```python
from build123d import *

# Parameters (mm, degrees)
F0_W     = 117.30712
F0_H     = 72.89958
F1_DEPTH = 25.4
F2_R     = 5.08
F3_R     = 5.08
F4_W     = 25.4
F4_H     = 72.89958
F5_DEPTH = 101.6


with BuildPart() as f1:
    # F0 (on Top) → F1 (new body)
    with BuildSketch(Plane.XY):
        Rectangle(F0_W, F0_H)
    extrude(amount=F1_DEPTH)

    # F2
    f2_edges = [f1.edges().sort_by_distance(p)[0] for p in [
        (58.65356, 36.44979, 12.7),
    ]]
    fillet(f2_edges, radius=F2_R)

    # F3
    f3_edges = [f1.edges().sort_by_distance(p)[0] for p in [
        (-58.65356, 36.44979, 12.7),
    ]]
    fillet(f3_edges, radius=F3_R)

    # F4 (on face) → F5 (join)
    with BuildSketch(Plane.XY.offset(25.4)):
        with Locations((-45.95356, 0)):
            Rectangle(F4_W, F4_H)
        with Locations((45.95356, 0)):
            Rectangle(F4_W, F4_H)
    extrude(amount=F5_DEPTH)


solid = f1.part
```
CAD build for the part. Positions are in the model's coordinates, mm. A direction names the side the tool comes from. Round coordinates to 2 decimals unless told otherwise and drop trailing zeros. Order: outer loops, then holes, each group sorted by start corner. A loop starts at its lowest first (then second) coordinate and runs counter-clockwise, first axis right, second up. Notation, with made-up numbers: (-30.5, -4.5) - (-6.5, -4.5) arc R30 cw to (-6.5, 34.5) - close; hole circle Ø3 at (42.25, -29). An arc over 180 degrees is marked (long way). Use CSV: the item, a comma, the result in double quotes. Start each with the question number.
1) Pin check, flat tips, straight feed: pin 1 Ø1.5 at (x, y) = (-22, 4) entering from -Z; pin 2 Ø20 at (x, y) = (-7.5, -6) entering from +Z. Stop position of each tip, or through.
2) Wall check: L1, parallel to X at y = -4, z = 74.5; L2, parallel to Z at x = 15.5, y = 10.5. Give the ranges that are in metal, low to high. Write a range as [from, to].
3) Saw through at C-C (x = 30.5). List the corners of the cut face in (y, z), and give its area (3 significant figures).
4) Saw through at A-A (z = 89). List the corners of the cut face in (x, y), and give its area (3 significant figures).
5) Two-plate mould, pull along X, no slides. Class faces 4 (the cylindrical face through (57.205, 34.922, 12.878)), 5 (the flat face through (0, 1, 25.4)), 6 (the flat face through (-33.254, -1, 75)), 7 (the flat face through (-1, 36.45, 20)): pulls with the +X half, pulls with the -X half, needs draft (parallel to the pull), parting line crosses it, or undercut.
6) Saw through at B-B (y = 10). List the corners of the cut face in (x, z).
7) Tool access for faces 1 (the flat face through (33.254, -1, 75)), 2 (the flat face through (57.4, 35.4, 25.4)), 3 (the cylindrical face through (-57.13, 35, 12.88)): list every direction of +Z, -Z, +X, -X, +Y, -Y with a clear straight run to the whole face (end or side of a thin tool).
Values follow:
1,pin 1,"stops at z = 0"
1,pin 2,"stops at z = 25.4"
2,L1,"x = [-58.65, -33.25], [33.25, 58.65]"
2,L2,"z = [0, 25.4]"
3,outline,"(-36.45, 0) - (36.45, 0) - (36.45, 25.4) - (-36.45, 25.4) - close"
3,area,"1,850 mm2"
4,outline,"(-58.65, -36.45) - (-33.25, -36.45) - (-33.25, 36.45) - (-58.65, 36.45) - close; (33.25, -36.45) - (58.65, -36.45) - (58.65, 36.45) - (33.25, 36.45) - close"
4,area,"3,700 mm2"
5,face 4,"pulls with the +X half"
5,face 5,"undercut"
5,face 6,"undercut"
5,face 7,"needs draft"
6,outline,"(-58.65, 0) - (58.65, 0) - (58.65, 127) - (33.25, 127) - (33.25, 25.4) - (-33.25, 25.4) - (-33.25, 127) - (-58.65, 127) - close"
7,face 1,"+Z, +Y, -Y"
7,face 2,"-Z, +X, +Y"
7,face 3,"-Z, -X, +Y"
